Work out the finished part from the listing and answer in its coordinate system (mm). Coordinates: 2 decimals unless noted, no trailing zeros. Write each loop counter-clockwise with the first axis right and the second up, starting at its lowest first coordinate (ties: lowest second). Pieces come first, ordered by that corner, then holes. Notation, with made-up numbers: M 17,-20.75 L 70,-20.75 A25 cw 70,13.25 Z; hole C 37.25,63 d6. An arc over 180 degrees is marked long. Use CSV: the item, a comma, the result in double quotes.
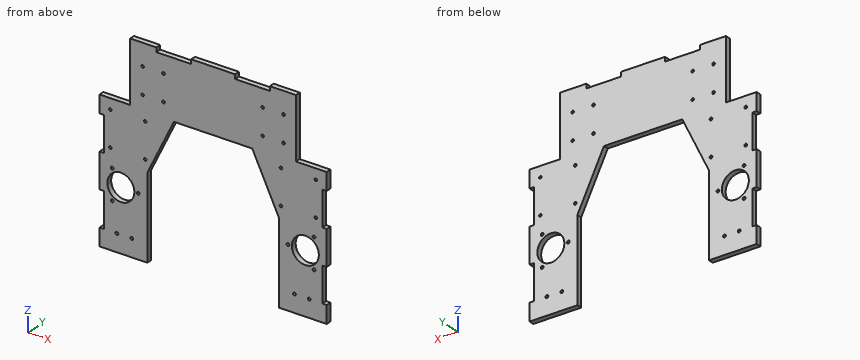
from build123d import *

# Parameters (mm, degrees)
BOSS_EXTRUDE1_DEPTH     = 6
SKETCH4_W               = 35.287296169
SKETCH4_H               = 70
CUT_EXTRUDE1_DEPTH      = 10
SKETCH8_W               = 55
SKETCH8_H               = 6
BOSS_EXTRUDE2_DEPTH     = 30
SKETCH10_W              = 5
SKETCH10_H              = 40
SKETCH10_W_2            = 40
SKETCH10_H_2            = 5
CUT_EXTRUDE2_DEPTH      = 10
SKETCH11_R              = 1.5
CUT_EXTRUDE3_DEPTH      = 10
SKETCH12_R              = 1.6
CUT_EXTRUDE4_DEPTH      = 27
SKETCH13_R              = 1.6
CUT_EXTRUDE5_DEPTH      = 39
SKETCH14_R              = 1.6
SKETCH14_R_2            = 1.5
CUT_EXTRUDE6_DEPTH      = 10
CUT_EXTRUDE7_DEPTH      = 436.116515514
CUT_EXTRUDE7_DEPTH_BACK = 15
SKETCH15_R              = 15.5
CUT_EXTRUDE8_DEPTH      = 436.116515514
CUT_EXTRUDE8_DEPTH_BACK = 436.116515514
SKETCH16_R              = 15.5


with BuildPart() as part:
    # Sketch3 → Boss-Extrude1 (new body)
    with BuildSketch(Plane(origin=(0, 0, 0), x_dir=(1, 0, 0), z_dir=(0, 1, 0))):
        Polygon((-85.132929843, 76.727687575), (-85.132929843, -123.272312425), (175.891655366, -123.272312425), (175.891655366, 76.727687575), (120.891655366, 76.727687575), (120.891655366, 11.727687575), (90.379362761, -51.272312425), (0.379362761, -51.272312425), (-30.132929843, 11.727687575), (-30.132929843, 76.727687575), align=None)
    extrude(amount=BOSS_EXTRUDE1_DEPTH)

    # Sketch4 → Cut-Extrude1 (cut)
    with BuildSketch(Plane(origin=(0, 6, 0), x_dir=(1, 0, 0), z_dir=(0, 1, 0))):
        with Locations((158.248007282, -88.272312425)):
            Rectangle(SKETCH4_W, SKETCH4_H)
        with Locations((-67.489281758, -88.272312425)):
            Rectangle(SKETCH4_W, SKETCH4_H)
    extrude(amount=-CUT_EXTRUDE1_DEPTH, mode=Mode.SUBTRACT)

    # Sketch8 → Boss-Extrude2 (add)
    with BuildSketch(Plane(origin=(0, 0, -76.727687575), x_dir=(-1, 0, 0), z_dir=(0, 0, -1))):
        with Locations((-148.391655366, 3)):
            Rectangle(SKETCH8_W, SKETCH8_H)
        with Locations((57.632929843, 3)):
            Rectangle(SKETCH8_W, SKETCH8_H)
    extrude(amount=BOSS_EXTRUDE2_DEPTH)

    # Sketch10 → Cut-Extrude2 (cut)
    with BuildSketch(Plane(origin=(0, 6, 0), x_dir=(1, 0, 0), z_dir=(0, 1, 0))):
        with Locations((-82.632929843, 66.727687575)):
            Rectangle(SKETCH10_W, SKETCH10_H)
        with Locations((-82.632929843, -13.272312425)):
            Rectangle(SKETCH10_W, SKETCH10_H)
        with Locations((173.391655366, -13.272312425)):
            Rectangle(SKETCH10_W, SKETCH10_H)
        with Locations((173.391655366, 66.727687575)):
            Rectangle(SKETCH10_W, SKETCH10_H)
        with Locations((0.154366326, -120.772312425)):
            Rectangle(SKETCH10_W_2, SKETCH10_H_2)
        with Locations((90.604359197, -120.772312425)):
            Rectangle(SKETCH10_W_2, SKETCH10_H_2)
    extrude(amount=-CUT_EXTRUDE2_DEPTH, mode=Mode.SUBTRACT)

    # Sketch11 → Cut-Extrude3 (cut)
    with BuildSketch(Plane(origin=(0, 0, 0), x_dir=(1, 0, 0), z_dir=(0, 1, 0))):
        with Locations(Location((-35.632929843, -68.272312425, 0), (0, 0, 90))):
            Circle(SKETCH11_R)
        with Locations(Location((-11.632929843, -68.272312425, 0), (0, 0, 90))):
            Circle(SKETCH11_R)
        with Locations(Location((-11.632929843, -98.272312425, 0), (0, 0, 90))):
            Circle(SKETCH11_R)
        with Locations(Location((-35.632929843, -98.272312425, 0), (0, 0, 90))):
            Circle(SKETCH11_R)
        with Locations(Location((102.391655366, -68.272312425, 0), (0, 0, 90))):
            Circle(SKETCH11_R)
        with Locations(Location((102.391655366, -98.272312425, 0), (0, 0, 90))):
            Circle(SKETCH11_R)
        with Locations(Location((126.391655366, -98.272312425, 0), (0, 0, 90))):
            Circle(SKETCH11_R)
        with Locations(Location((126.391655366, -68.272312425, 0), (0, 0, 90))):
            Circle(SKETCH11_R)
    extrude(amount=CUT_EXTRUDE3_DEPTH, mode=Mode.SUBTRACT)

    # Sketch12 → Cut-Extrude4 (cut)
    with BuildSketch(Plane(origin=(0, 0, 0), x_dir=(1, 0, 0), z_dir=(0, 1, 0))):
        with Locations(Location((138.891655366, 86.727687575, 0), (0, 0, 90))):
            Circle(SKETCH12_R)
        with Locations(Location((155.891655366, 86.727687575, 0), (0, 0, 90))):
            Circle(SKETCH12_R)
    extrude(amount=CUT_EXTRUDE4_DEPTH, mode=Mode.SUBTRACT)

    # Sketch13 → Cut-Extrude5 (cut)
    with BuildSketch(Plane(origin=(0, 0, 0), x_dir=(1, 0, 0), z_dir=(0, 1, 0))):
        with Locations(Location((-65.132929843, 86.727687575, 0), (0, 0, 90))):
            Circle(SKETCH13_R)
        with Locations(Location((-48.132929843, 86.727687575, 0), (0, 0, 90))):
            Circle(SKETCH13_R)
    extrude(amount=CUT_EXTRUDE5_DEPTH, mode=Mode.SUBTRACT)

    # Sketch14 → Cut-Extrude6 (cut)
    with BuildSketch(Plane(origin=(0, 0, 0), x_dir=(1, 0, 0), z_dir=(0, 1, 0))):
        with Locations(Location((-70.632929843, 54.227687575, 0), (0, 0, 90))):
            Circle(SKETCH14_R)
        with Locations(Location((-40.632929843, 36.907179499, 0), (0, 0, 90))):
            Circle(SKETCH14_R)
        with Locations(Location((-70.632929843, 19.586671424, 0), (0, 0, 90))):
            Circle(SKETCH14_R)
        with Locations(Location((-72.632929843, -1.247312425, 0), (0, 0, 90))):
            Circle(SKETCH14_R_2)
        with Locations(Location((-32.632929843, -1.247312425, 0), (0, 0, 90))):
            Circle(SKETCH14_R_2)
        with Locations(Location((-32.632929843, -41.247312425, 0), (0, 0, 90))):
            Circle(SKETCH14_R_2)
        with Locations(Location((-72.632929843, -41.247312425, 0), (0, 0, 90))):
            Circle(SKETCH14_R_2)
        with Locations(Location((163.391655366, -41.247312425, 0), (0, 0, 90))):
            Circle(SKETCH14_R_2)
        with Locations(Location((123.391655366, -41.247312425, 0), (0, 0, 90))):
            Circle(SKETCH14_R_2)
        with Locations(Location((123.391655366, -1.247312425, 0), (0, 0, 90))):
            Circle(SKETCH14_R_2)
        with Locations(Location((163.391655366, -1.247312425, 0), (0, 0, 90))):
            Circle(SKETCH14_R_2)
        with Locations(Location((161.391655366, 19.586671424, 0), (0, 0, 90))):
            Circle(SKETCH14_R)
        with Locations(Location((131.391655366, 36.907179499, 0), (0, 0, 90))):
            Circle(SKETCH14_R)
        with Locations(Location((161.391655366, 54.227687575, 0), (0, 0, 90))):
            Circle(SKETCH14_R)
    extrude(amount=CUT_EXTRUDE6_DEPTH, mode=Mode.SUBTRACT)

    # Sketch15 → Cut-Extrude7 (cut, two sides: drawn at the far end of the back side and taken through both)
    with BuildSketch(Plane(origin=(-65.954618325, -135.210856749, -209.738582158), x_dir=(1, 0, 0), z_dir=(0, 1, 0)).offset(-CUT_EXTRUDE7_DEPTH_BACK)):
        with Locations(Location((5.321688481, -172.831402658, 0), (0, 0, 270))):
            Circle(SKETCH15_R)
    extrude(amount=CUT_EXTRUDE7_DEPTH + CUT_EXTRUDE7_DEPTH_BACK, mode=Mode.SUBTRACT)

    # Sketch16 → Cut-Extrude8 (cut, two sides: drawn at the far end of the back side and taken through both)
    with BuildSketch(Plane(origin=(-65.954618325, -135.210856749, -209.738582158), x_dir=(1, 0, 0), z_dir=(0, 1, 0)).offset(-CUT_EXTRUDE8_DEPTH_BACK)):
        with Locations(Location((217.346273691, -172.831402658, 0), (0, 0, 90))):
            Circle(SKETCH16_R)
    extrude(amount=CUT_EXTRUDE8_DEPTH + CUT_EXTRUDE8_DEPTH_BACK, mode=Mode.SUBTRACT)


solid = part.part
Item 1: Consider probe 1 along X at (y, z) = (1.7, -74); probe 2 along Z at (x, y) = (131.5, 4); probe 3 along Z at (x, y) = (131, 5.1). Determine where each line is inside the solid, lowest interval first.
Answer:
probe 1,"x = -80.13 to -30.13, 120.89 to 170.89"
probe 2,"z = -106.73 to -38.5, -35.31 to 123.27"
probe 3,"z = -106.73 to -38.46, -35.36 to 123.27"
Item 2: Given pin 1 (3.5 mm diameter, centred on x = -35.63, z = 98.27, fed in from -Y); pin 2 (3 mm diameter, centred on y = 2, z = 97.5, fed in from -X), each flat-ended and moving along its own axis, determine where each tip first touches the part or whether it passes through.
Answer:
pin 1,"stops at y = 0"
pin 2,"stops at x = -49.85"
Item 3: The part is cut by section A-A (z = -79). Write down the section's boundary in (x, y).
Answer:
outline,"M -80.13,0 L -30.13,0 L -30.13,6 L -80.13,6 Z; M 120.89,0 L 170.89,0 L 170.89,6 L 120.89,6 Z"
Item 4: The part is cut by section C-C (x = 60). Write down the section's boundary in (y, z), then the cut area to 3 significant figures.
Answer:
outline,"M 0,51.27 L 6,51.27 L 6,123.27 L 0,123.27 Z"
area,"432 mm2"
Item 5: The part is cut by section B-B (z = -30). Write down the section's boundary in (x, y), then the cut area to 3 significant figures.
Answer:
outline,"M -85.13,0 L -74.51,0 L -74.51,6 L -85.13,6 Z; M -46.76,0 L -30.13,0 L -30.13,6 L -46.76,6 Z; M 120.89,0 L 137.52,0 L 137.52,6 L 120.89,6 Z; M 165.27,0 L 175.89,0 L 175.89,6 L 165.27,6 Z"
area,"327 mm2"
Item 6: The part is cut by section D-D (z = 17). Write down the section's boundary in (x, y), then the cut area to 3 significant figures.
Answer:
outline,"M -80.13,0 L -16.22,0 L -16.22,6 L -80.13,6 Z; M 106.98,0 L 170.89,0 L 170.89,6 L 106.98,6 Z"
area,"767 mm2"
